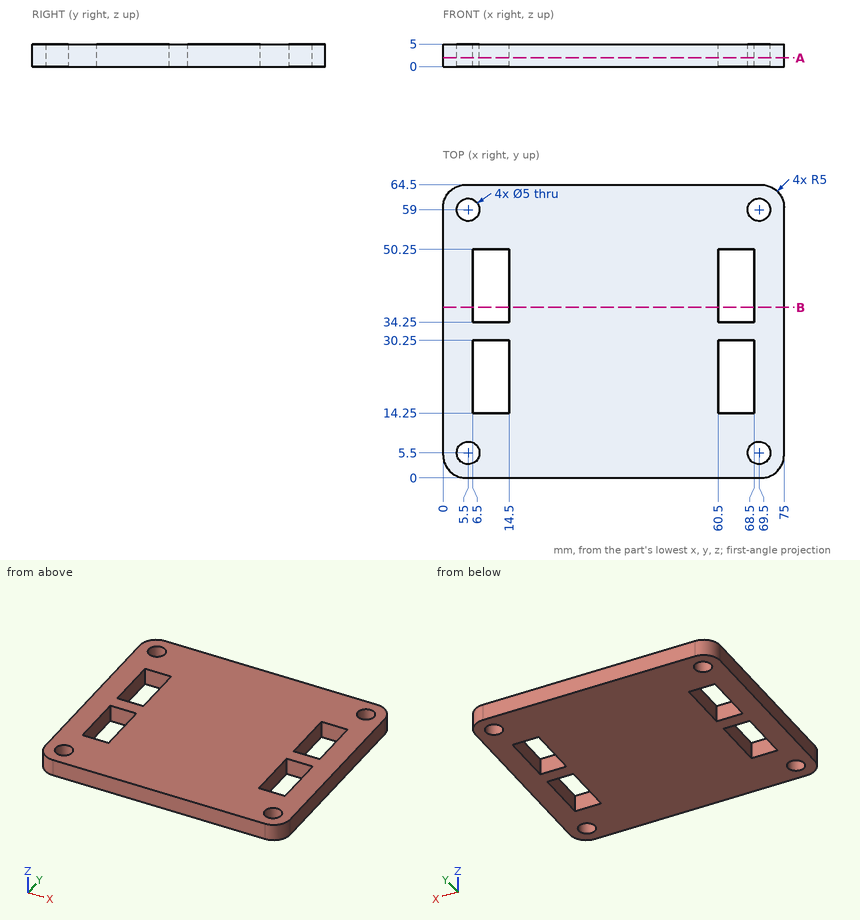
Drawing for the job (mm, zero at the part's lowest x, y, z). Coordinates: 2 decimals unless noted, no trailing zeros. Order: outer loops, then holes, each group sorted by start corner. A loop starts at its lowest first (then second) coordinate and runs counter-clockwise, first axis right, second up. Notation, with made-up numbers: (-2.75, 80) -> (15.25, 80) arc R24 cw to (15.25, 102) -> close; hole circle Ø10 at (7, -19.75). An arc over 180 degrees is marked (long way). Answer in a Markdown table with one row per item.
1) Band-saw the part on A-A (z = 1.95). Give the number of separate pieces and of enclosed holes in the cut face, and give its area (3 significant figures).
Check values:
| item | result |
|---|---|
| separate pieces | 1 |
| enclosed holes | 8 |
| area | 4,230 mm2 |
2) Drill centre lines: line 1 (X direction, y = 26.5, z = 0.35); line 2 (Y direction, x = 5.5, z = 3.45); line 3 (Y direction, x = 61, z = 1.6). Where is each one in solid material? Low to high.
Check values:
| item | result |
|---|---|
| line 1 | 0 to 6.5, 14.5 to 60.5, 68.5 to 75 |
| line 2 | 0 to 3, 8 to 56.5, 61.5 to 64.5 |
| line 3 | 0 to 14.25, 30.25 to 34.25, 50.25 to 64.5 |
3) Band-saw the part on B-B (y = 37.5). List the corners of the cut face in (x, z), and give its area (3 significant figures).
Check values:
| item | result |
|---|---|
| outline | (0, 0) -> (6.5, 0) -> (6.5, 5) -> (0, 5) -> close; (14.5, 0) -> (60.5, 0) -> (60.5, 5) -> (14.5, 5) -> close; (68.5, 0) -> (75, 0) -> (75, 5) -> (68.5, 5) -> close |
| area | 295 mm2 |
